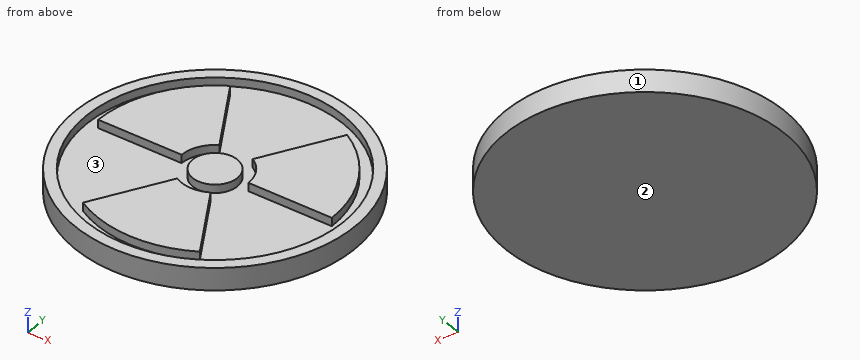
Autodesk Fusion 360 part; units mm, degrees
sketch "Sketch2" plane through (0, 0, 0) normal (0, 0, 1) x (1, 0, 0)
  circle A0 centre (0, 0) radius 25
  dimension "d3" = 50
extrude "Extrude2" add sketch "Sketch2" along normal blind 2.5
sketch "Sketch3" plane through (0, 0, 2.5) normal (0, 0, 1) x (-1, 0, 0)
  circle A0 centre (0, 0) radius 25
  circle A1 centre (0, 0) radius 23
  circle A2 centre (0, 0) radius 21
  circle A3 centre (0, 0) radius 4
  line L0 (6, 0) -> (3, 5.1962) construction
  line L1 (3, 5.1962) -> (-3, 5.1962) construction
  line L2 (-3, 5.1962) -> (-6, 0) construction
  line L3 (-6, 0) -> (-3, -5.1962) construction
  line L4 (-3, -5.1962) -> (3, -5.1962) construction
  line L5 (3, -5.1962) -> (6, 0) construction
  line L6 (-3, -5.1962) -> (-10.5, -18.1865)
  line L7 (-6, 0) -> (-21, 0)
  line L8 (-3, 5.1962) -> (-10.5, 18.1865)
  line L9 (3, 5.1962) -> (10.5, 18.1865)
  line L10 (6, 0) -> (21, 0)
  line L11 (3, -5.1962) -> (10.5, -18.1865)
  line L12 (21, 0) -> (10.5, -18.1865) construction
  line L13 (-10.5, -18.1865) -> (-21, 0) construction
  line L14 (-10.5, 18.1865) -> (-21, 0) construction
  line L15 (-10.5, -18.1865) -> (10.5, -18.1865) construction
  line L16 (21, 0) -> (10.5, 18.1865) construction
  circle A4 centre (0, 0) radius 6
  dimension "d6" = -2
  dimension "d7" = -4
  dimension "d8" = 8
  dimension "d9" = 6
extrude "Extrude3" add sketch "Sketch3" along normal blind 1.5 contours A0 | A2 L10 L11 A4 | A2 L8 L9 A4 | A2 L6 L7 A4
extrude "Extrude4" add sketch "Sketch3" along normal blind 1.5 contours A3
Input: part model. Units: mm. Frame: model coordinates. Face numbers are marked on the shaded views. Give positions to 0.01 mm unless a question says otherwise; leave off trailing zeros. Loops run counter-clockwise (first coordinate to the right, second up) from the corner with the lowest first, then second, coordinate; pieces in that order, holes last.
1) Line query: L1, parallel to Y at x = 0, z = 3.5; L2, parallel to X at y = -9.5, z = 3.6; L3, parallel to Z at x = -1, y = 21. Output: solid intervals per line, ascending.
A:
L1: y = -25 to -23, -21 to -6, -4 to 4, 23 to 25
L2: x = -23.12 to -20.95, -5.48 to 5.48, 20.95 to 23.12
L3: z = 0 to 2.5
2) Mould query, pull axis Y, two halves, no side actions, for the marked faces 1, 2 and 3. Classes: released by +Y, released by -Y, zero draft, split by the parting line, or undercut.
A:
face 1: split by the parting line
face 2: zero draft
face 3: undercut
3) Section query B-B on z = 0.6. Return the cut outline in (x, y).
A:
outline: circle Ø50 at (0, 0)
4) Section query A-A on z = 3.3. Return the cut outline in (x, y).
A:
outline: circle Ø50 at (0, 0); (-21, 0) - (-6, 0) arc R6 cw to (-3, 5.2) - (-10.5, 18.19) arc R21 ccw to start; (-10.5, -18.19) arc R21 ccw to (10.5, -18.19) - (3, -5.2) arc R6 cw to (-3, -5.2) - close; circle Ø8 at (0, 0); (3, 5.2) arc R6 cw to (6, 0) - (21, 0) arc R21 ccw to (10.5, 18.19) - close; hole circle Ø46 at (0, 0)
5) Contact query for flat-ended pins moving along their axis: pin 1 (1.2 mm diameter, centred on x = -14.5, z = 3, fed in from -Y); pin 2 (1.2 mm diameter, centred on x = 16.5, z = 3.5, fed in from -Y); pin 3 (1 mm diameter, centred on y = 12.5, z = 0.5, fed in from -X). Output: stop coordinate, or through.
A:
pin 1: stops at y = -20.78
pin 2: stops at y = -19.29
pin 3: stops at x = -21.93
